Autodesk Inventor part; units mm, degrees
ref_plane "YZ Plane" through (0, 0, 0) normal (1, 0, 0) x (0, 1, 0)
ref_plane "XZ Plane" through (0, 0, 0) normal (0, 1, 0) x (-1, 0, 0)
ref_plane "XY Plane" through (0, 0, 0) normal (0, 0, 1) x (1, 0, 0)
sketch "Sketch1" plane through (0, 0, 0) normal (0, 1, 0) x (-1, 0, 0)
  line L0 (-10, 21) -> (10, 21)
  line L1 (10, 21) -> (10, -21)
  line L2 (10, -21) -> (-10, -21)
  line L3 (-10, -21) -> (-10, 21)
  line L4 (-10, 21) -> (10, -21) construction
  line L5 (10, 21) -> (-10, -21) construction
  point P0 (0, 0)
  dimension "d0" = 20
  dimension "d1" = 42
extrude "Extrusion1" add sketch "Sketch1" along normal blind 3
sketch "Sketch2" plane through (10, 0, 21) normal (1, 0, 0) x (0, 0, -1)
  line L0 (0, 0) -> (10, 0)
  line L1 (10, 0) -> (10, 45)
  line L2 (10, 45) -> (0, 45)
  line L3 (0, 45) -> (0, 0)
  line L4 (42, 0) -> (0, 0)
  line L5 (42, 0) -> (32, 0)
  line L6 (32, 0) -> (32, 45)
  line L7 (32, 45) -> (42, 45)
  line L8 (42, 45) -> (42, 0)
  point P0 (21, 0)
  dimension "d4" = 10
  dimension "d5" = 45
  dimension "d6" = 10
  dimension "d7" = 45
extrude "Extrusion2" add sketch "Sketch2" along normal blind 3
sketch "Sketch3" plane through (13, 0, 21) normal (1, 0, 0) x (0, 0, -1)
  circle A0 centre (5, 40) radius 1.5
  circle A1 centre (5, 8) radius 1.5
  point P0 (21, 0)
  dimension "d10" = 3
  dimension "d11" = 3
extrude "Extrusion3" cut sketch "Sketch3" against normal blind 3
mirror "Mirror1" about plane through (0, 0, 0) normal (0, 0, 1) of "Extrusion3"
sketch "Sketch5" plane through (0, 3, 0) normal (0, 1, 0) x (1, 0, 0)
  circle A0 centre (0, -11) radius 2
  circle A1 centre (0, 11) radius 2
  point P0 (0, 0)
  dimension "d18" = 4
  dimension "d19" = 4
extrude "Extrusion5" cut sketch "Sketch5" against normal blind 3
sketch "Sketch6" plane through (0, 3, 0) normal (0, 1, 0) x (1, 0, 0)
  point P0 (0, 0)
thicken "Thicken1" operation add thickness 17 both sides no extend neighbours yes toward (-1, 0, 0) faces at (-10, 1, -7)
properties part number "vertical_axis_motor_metal_holder" material "Aluminum 6061"
Here's how the part is built. I have some questions about the finished solid (model axes, mm). A direction names the side the tool comes from. Coordinates: 2 decimals unless noted, no trailing zeros. Write each loop counter-clockwise with the first axis right and the second up, starting at its lowest first coordinate (ties: lowest second). Pieces come first, ordered by that corner, then holes. Notation, with made-up numbers: (60, 6) - (68, 6) arc R32 cw to (68, 34) - close; hole circle Ø6 at (8.5, 12.25). An arc over 180 degrees is marked (long way). One line per item, written item: value.
1) We'd pull the mould along Y, two halves only. Please class faces 1 (the cylindrical face through (11.5, 8.9, -17.2)), 2 (the flat face through (-8, 3, 0)), 3 (the flat face through (-27, 1, 0)): pulls with the +Y half, pulls with the -Y half, needs draft (parallel to the pull), parting line crosses it, or undercut.
Model answer:
face 1: undercut
face 2: pulls with the +Y half
face 3: needs draft
2) On a 3-axis mill with a long thin cutter (end or side, diameter ignored), from which of +Z, -Z, +X, -X, +Y, -Y can I reach the whole of each face in a straight line? I mean faces 4 (the flat face through (10, 1, 0)), 5 (the cylindrical face through (0, 2, -13)), 6 (the flat face through (10, 24, 16)). Say none if no direction works.
Model answer:
face 4: +X, +Y, -Y
face 5: +Y, -Y
face 6: +Z, -Z, -X, +Y
3) I'm going to push flat-ended pins straight in: P1, Ø8, axis at y = 38.5, z = 5.5, coming from the -X side; P2, Ø4.5, axis at x = 0, z = -11, coming from the +Y side; P3, Ø3, axis at y = 25, z = 18, coming from the -X side; P4, Ø0.9, axis at y = 2, z = 0, coming from the +X side. Where does each tip first touch, or does it pass through?
Model answer:
P1: passes through
P2: stops at y = 3
P3: stops at x = 10
P4: stops at x = 10
4) I need wall thicknesses on line 1 along Y through (x, z) = (11.2, -16); line 2 along Z through (x, y) = (0, 0.7); line 3 along Y through (x, z) = (-14, -5.5). Which ranges of each line are inside material? Lowest first, please.
Model answer:
line 1: y = 0 to 6.5, 9.5 to 38.5, 41.5 to 45
line 2: z = -21 to -13, -9 to 9, 13 to 21
line 3: y = 0 to 3
5) Suppose I cut it at C-C on x = 0. Write out the boundary of the cut face in (y, z).
Model answer:
outline: (0, -21) - (3, -21) - (3, -13) - (0, -13) - close; (0, -9) - (3, -9) - (3, 9) - (0, 9) - close; (0, 13) - (3, 13) - (3, 21) - (0, 21) - close
6) Suppose I cut it at A-A on y = 40. Write out the boundary of the cut face in (x, z).
Model answer:
outline: (10, -21) - (13, -21) - (13, -17.5) - (10, -17.5) - close; (10, -14.5) - (13, -14.5) - (13, -11) - (10, -11) - close; (10, 11) - (13, 11) - (13, 14.5) - (10, 14.5) - close; (10, 17.5) - (13, 17.5) - (13, 21) - (10, 21) - close
7) Suppose I cut it at B-B on z = -16. Write out the boundary of the cut face in (x, y).
Model answer:
outline: (-27, 0) - (13, 0) - (13, 6.5) - (10, 6.5) - (10, 3) - (-27, 3) - close; (10, 9.5) - (13, 9.5) - (13, 38.5) - (10, 38.5) - close; (10, 41.5) - (13, 41.5) - (13, 45) - (10, 45) - close
8) Suppose I cut it at D-D on y = 30. Write out the boundary of the cut face in (x, z).
Model answer:
outline: (10, -21) - (13, -21) - (13, -11) - (10, -11) - close; (10, 11) - (13, 11) - (13, 21) - (10, 21) - close
